from build123d import *

# Parameters (mm, degrees)
F0_W     = 63.5
F0_H     = 101.6
F1_DEPTH = 6.35
F2_R     = 4.7625
F3_DEPTH = 69.85
F4_W     = 6.35
F4_H     = 25.4
F5_DEPTH = 44.45


with BuildPart() as f1:
    # F0 (on Top) → F1 (new body)
    with BuildSketch(Plane.XY):
        Rectangle(F0_W, F0_H)
    extrude(amount=F1_DEPTH)

    # F2 (on face) → F3 (join)
    with BuildSketch(Plane.XY.offset(6.35)):
        Circle(F2_R)
    extrude(amount=F3_DEPTH)

    # F4 (on face) → F5 (join)
    with BuildSketch(Plane.XY.offset(6.35)):
        with Locations((-28.575, -12.7)):
            Rectangle(F4_W, F4_H)
    extrude(amount=F5_DEPTH)


solid = f1.part
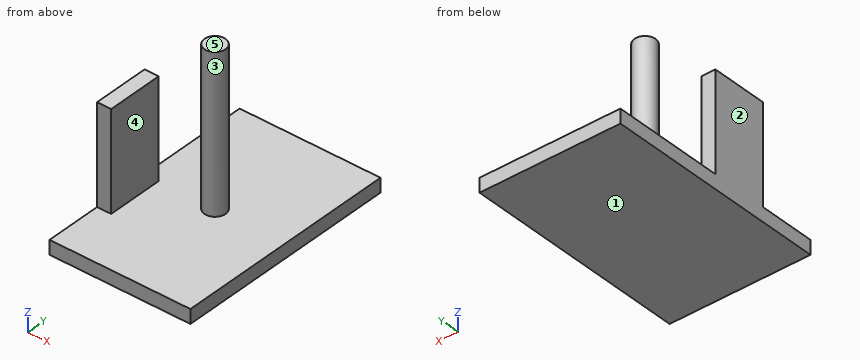
Verification items for the finished model (mm, model axes). Face numbers are marked on the shaded views. A direction names the side the tool comes from. Give positions to 0.01 mm unless a question says otherwise; leave off trailing zeros. Order: outer loops, then holes, each group sorted by start corner. A loop starts at its lowest first (then second) coordinate and runs counter-clockwise, first axis right, second up. Notation, with made-up numbers: M 65.25,63 L 78.25,63 A11 cw 78.25,81 Z; hole C -27,89.25 d2. An arc over 180 degrees is marked long. Use one line per item in the form item = value. Start each with the question number.
Q1. Mould release check, pull along X, two halves, no side actions. Record for the marked faces 1, 2 and 3: +X half, -X half, draft (parallel to the pull), parting line (faces both ways), or undercut.
Q2. Scan lines: line 1 along Z through (x, y) = (-25.5, 32.5); line 2 along Y through (x, z) = (0, 55); line 3 along Y through (x, z) = (-4, 50). Record each from-to range of solid material in increasing order. Write a range as [from, to].
Q3. Section check A-A (x = 0). Enter the section's corners in (y, z).
Q4. Section check C-C (y = -24). Enter the section's corners in (x, z), then the cut area to 3 significant figures.
Q5. Go/stop test with flat-tipped pins: pin 1 Ø6 at (x, z) = (-24.5, 35) entering from -Y; pin 2 Ø3 at (x, y) = (-22.5, -17) entering from +Z; pin 3 Ø4 at (x, y) = (-23, -32.5) entering from -Z; pin 4 Ø5 at (x, z) = (-3.5, 10.5) entering from +Y. Record where each tip stops, or that it passes through.
Q6. Section check D-D (z = 60). Enter the section's corners in (x, y) (1 decimal), then the cut area to 3 significant figures.
Q7. Access from +Z, -Z, +X, -X, +Y, -Y to the whole of each face (thin tool, end or side, straight path). Record for the marked faces 4 and 5.
Evaluation:
q1.face_1 = draft
q1.face_2 = -X half
q1.face_3 = undercut
q2.line_1 = [0, 6.35]
q2.line_2 = [-4.76, 4.76]
q2.line_3 = [-2.58, 2.58]
q3.outline = M -50.8,0 L 50.8,0 L 50.8,6.35 L 4.76,6.35 L 4.76,76.2 L -4.76,76.2 L -4.76,6.35 L -50.8,6.35 Z
q4.outline = M -31.75,0 L 31.75,0 L 31.75,6.35 L -25.4,6.35 L -25.4,50.8 L -31.75,50.8 Z
q4.area = 685 mm2
q5.pin_1 = -25.4
q5.pin_2 = 6.35
q5.pin_3 = 0
q5.pin_4 = 4.66
q6.outline = C 0,0 d9.5
q6.area = 71.3 mm2
q7.face_4 = +Z, +Y, -Y
q7.face_5 = +Z, +X, -X, +Y, -Y
